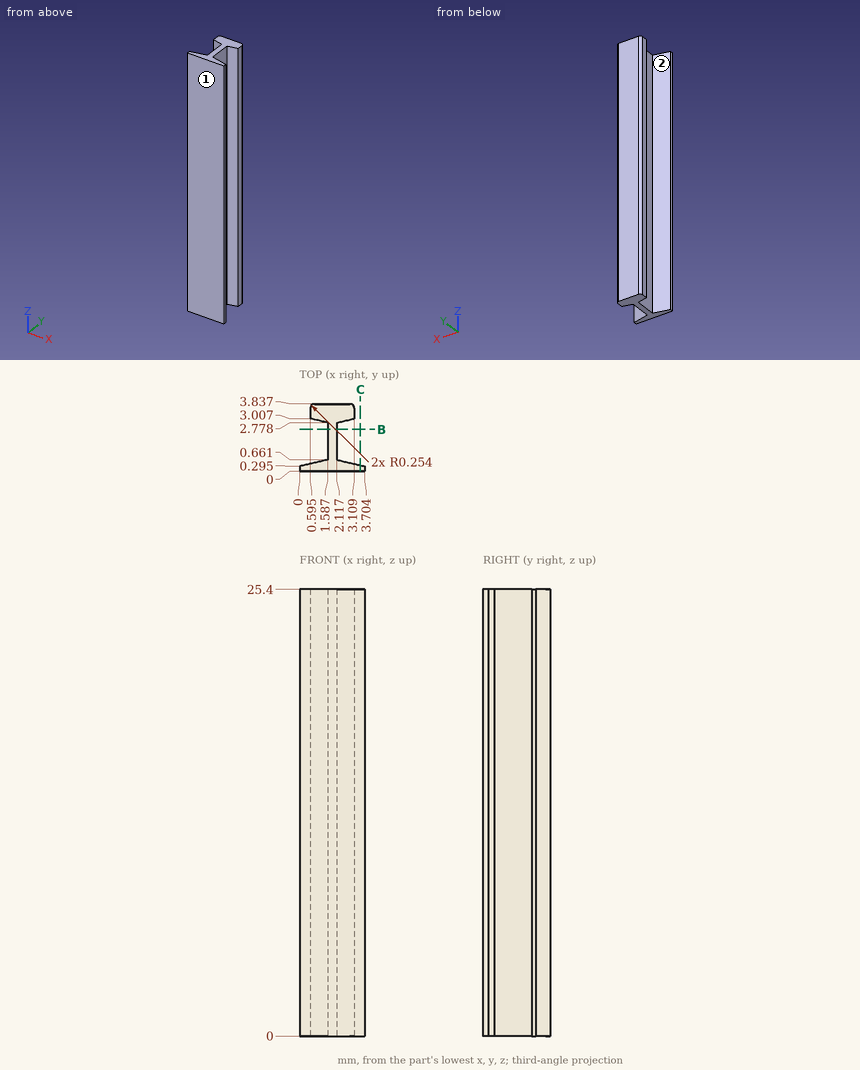
Here's the drawing with two shaded views (mm, measured from the low corner). I have some questions. A direction names the side the tool comes from. Coordinates: 2 decimals unless noted, no trailing zeros. Write each loop counter-clockwise with the first axis right and the second up, starting at its lowest first coordinate (ties: lowest second). Pieces come first, ordered by that corner, then holes. Notation, with made-up numbers: (33.5, -8.5) -> (77.5, -8.5) arc R26 cw to (77.5, 10.5) -> close; hole circle Ø5 at (-28.5, 47). An arc over 180 degrees is marked (long way). Use a Markdown table: item, result. Add a question column.
(1) Please list where these lines run through material, in increasing order: line 1 (X direction, y = 2.7, z = 2); line 2 (Y direction, x = 1.25, z = 4) (1 decimal); line 3 (Y direction, x = 1.55, z = 4).
(2) I'm going to push flat-ended pins straight in: P1, Ø1, axis at x = 1.5, y = 1.5, coming from the +Z side; P2, Ø1.1, axis at y = 1.5, z = 15.5, coming from the -X side; P3, Ø0.6, axis at y = 2, z = 18.5, coming from the +X side; P4, Ø0.6, axis at y = 3.5, z = 14.5, coming from the +X side. Where does each tip first touch, or does it pass through?
(3) If we section it at B-B, the plane y = 2.4: Write out the boundary of the cut face in (x, z).
(4) For the marked faces 1 and 2, which set-ups out of +Z, -Z, +X, -X, +Y, -Y let a thin tool reach every point of the face, with its end or its side?
(5) If we section it at C-C, the plane x = 3.45: Write out the boundary of the cut face in (y, z).
Outcome:
| question | item | result |
|---|---|---|
| 1 | line 1 | x = 1.59 to 2.12 |
| 1 | line 2 | y = 0 to 0.6, 2.9 to 3.8 |
| 1 | line 3 | y = 0 to 0.65, 2.79 to 3.84 |
| 2 | P1 | stops at z = 25.4 |
| 2 | P2 | stops at x = 1.59 |
| 2 | P3 | stops at x = 2.12 |
| 2 | P4 | stops at x = 3.11 |
| 3 | outline | (1.59, 0) -> (2.12, 0) -> (2.12, 25.4) -> (1.59, 25.4) -> close |
| 4 | face 1 | +Z, -Z, +X, -X, -Y |
| 4 | face 2 | +Z, -Z, -X |
| 5 | outline | (0, 0) -> (0.35, 0) -> (0.35, 25.4) -> (0, 25.4) -> close |
